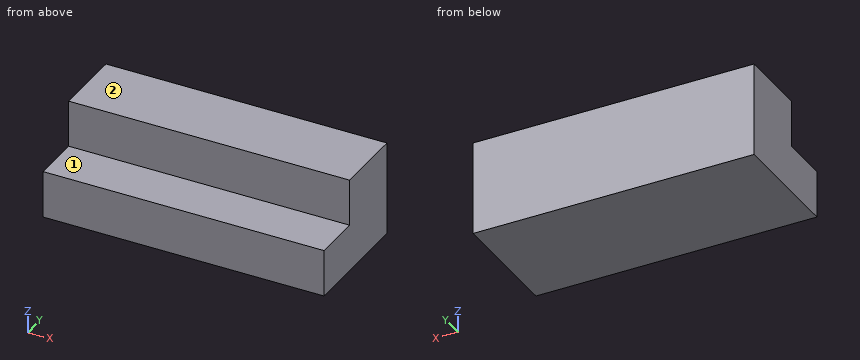
from build123d import *

# Parameters (mm, degrees)
F1_DEPTH = 76.2
F2_DEPTH = 76.2


with BuildPart() as f1:
    # F0 (on Right) → F1 (new body)
    with BuildSketch(Plane.YZ):
        Polygon((-38.252957, 0), (0, 0), (25.933029, 0), (25.933029, 50.999308), (-12.166971, 50.999308), (-12.166971, 25.599308), (-38.252957, 25.599308), align=None)
    extrude(amount=F1_DEPTH)

    # F1_face (on face) → F2 (join)
    with BuildSketch(Plane(origin=(0, -1.325449, 22.251354), x_dir=(0, 1, 0), z_dir=(-1, 0, 0))):
        Polygon((-36.927508, 22.251354), (-36.927508, -3.347954), (-10.841522, -3.347954), (-10.841522, -28.747954), (27.258478, -28.747954), (27.258478, 22.251354), align=None)
    extrude(amount=F2_DEPTH)


solid = f1.part
Read the model definition and answer for the solid it produces. Units are mm, in the model's axes. Face numbers are marked on the shaded views. A direction names the side the tool comes from. Coordinates: 2 decimals unless noted, no trailing zeros. Write each loop counter-clockwise with the first axis right and the second up, starting at its lowest first coordinate (ties: lowest second). Pieces come first, ordered by that corner, then holes. Notation, with made-up numbers: (75.25, 58.25) -> (105.25, 58.25) arc R19 cw to (105.25, 68.25) -> close; hole circle Ø4 at (50.25, -11). An arc over 180 degrees is marked (long way). Return JSON: item names as keys, results as strings.
(1) Which of the six approach directions +Z, -Z, +X, -X, +Y, -Y give full straight-line access (tool end or side, diameter ignored) to the marked faces 1 and 2?
Answers below:
{"face 1": "+Z, +X, -X, -Y", "face 2": "+Z, +X, -X, +Y, -Y"}
(2) Each of these flat-tipped pins is pushed along its axis until it touches: P1, Ø8, axis at x = 1.5, y = -31, coming from the +Z side; P2, Ø1, axis at x = -44, y = -13, coming from the -Z side; P3, Ø20.5, axis at x = 2.5, z = 44.5, coming from the -Y side. Where does it stop, or does it pass through?
Answers below:
{"P1": "z = 25.6", "P2": "z = 0", "P3": "y = -12.17"}
(3) The part is cut by section A-A on x = 47. Give the vertices of the cut face in (y, z).
Answers below:
{"outline": "(-38.25, 0) -> (25.93, 0) -> (25.93, 51) -> (-12.17, 51) -> (-12.17, 25.6) -> (-38.25, 25.6) -> close"}
(4) The part is cut by section C-C on z = 38. Give the vertices of the cut face in (x, y).
Answers below:
{"outline": "(-76.2, -12.17) -> (76.2, -12.17) -> (76.2, 25.93) -> (-76.2, 25.93) -> close"}
(5) The part is cut by section B-B on y = -25.5. Give the vertices of the cut face in (x, z), then the cut area to 3 significant figures.
Answers below:
{"outline": "(-76.2, 0) -> (76.2, 0) -> (76.2, 25.6) -> (-76.2, 25.6) -> close", "area": "3,900 mm^2"}
(6) Consider line 1 along Z through (x, y) = (-68, -15.5); line 2 along Y through (x, z) = (12.5, 47.5). Determine where each line is inside the solid, lowest interval first. Write a range as from..to.
Answers below:
{"line 1": "0..25.6", "line 2": "-12.17..25.93"}
